Here's how the part is built. I have some questions about the finished solid (model axes, mm). A direction names the side the tool comes from. Round coordinates to 2 decimals unless told otherwise and drop trailing zeros. Loops run counter-clockwise (first coordinate to the right, second up) from the corner with the lowest first, then second, coordinate; pieces in that order, holes last. Notation, with made-up numbers: M 45.25,9 L 102.25,9 A28 ccw 102.25,39 Z; hole C 78,74 d11. An arc over 180 degrees is marked long. Use a Markdown table: item, result.
```python
from build123d import *

# Parameters (mm, degrees)
F1_R      = 11
F1_R_2    = 2.25
F2_DEPTH  = 2
F1_R_3    = 1.75
F3_DEPTH  = 8
F4_DEPTH  = 4.5
F5_DEPTH  = 20
F7_DEPTH  = 24
F9_DEPTH  = 8
F10_R     = 4
F11_DEPTH = 1


with BuildPart() as f2:
    # F1 (on Top) → F2 (new body)
    with BuildSketch(Plane.XY):
        Circle(F1_R)
        Circle(F1_R_2, mode=Mode.SUBTRACT)
    extrude(amount=F2_DEPTH)

    # F1 (on Top) → F3 (join)
    with BuildSketch(Plane.XY):
        Polygon((21.15, 17.15), (17.15, 21.15), (-17.15, 21.15), (-21.15, 17.15), (-21.15, -17.15), (-17.15, -21.15), (17.15, -21.15), (21.15, -17.15), align=None)
        with Locations((-15.5, -15.5)):
            Circle(F1_R_3, mode=Mode.SUBTRACT)
        with Locations((15.5, -15.5)):
            Circle(F1_R_3, mode=Mode.SUBTRACT)
        with Locations((-15.5, 15.5)):
            Circle(F1_R_3, mode=Mode.SUBTRACT)
        Circle(F1_R, mode=Mode.SUBTRACT)
        with Locations((15.5, 15.5)):
            Circle(F1_R_3, mode=Mode.SUBTRACT)
        Circle(F1_R)
        Circle(F1_R_2, mode=Mode.SUBTRACT)
        Circle(F1_R_2)
        with Locations((15.5, -15.5)):
            Circle(F1_R_3)
        with Locations((-15.5, -15.5)):
            Circle(F1_R_3)
        with Locations((-15.5, 15.5)):
            Circle(F1_R_3)
        with Locations((15.5, 15.5)):
            Circle(F1_R_3)
    extrude(amount=-F3_DEPTH)

    # F1 (on Top) → F4 (cut)
    with BuildSketch(Plane.XY):
        with Locations((-15.5, 15.5)):
            Circle(F1_R_3)
        with Locations((15.5, 15.5)):
            Circle(F1_R_3)
        with Locations((15.5, -15.5)):
            Circle(F1_R_3)
        with Locations((-15.5, -15.5)):
            Circle(F1_R_3)
    extrude(amount=-F4_DEPTH, mode=Mode.SUBTRACT)

    # F1 (on Top) → F5 (join)
    with BuildSketch(Plane.XY):
        Circle(F1_R_2)
    extrude(amount=F5_DEPTH)

    # F6 (on face) → F7 (join)
    with BuildSketch(Plane(origin=(0, 0, -8), x_dir=(1, 0, 0), z_dir=(0, 0, -1))):
        Polygon((-13.15, 21.15), (-21.15, 13.15), (-21.15, -13.15), (-13.15, -21.15), (13.15, -21.15), (21.15, -13.15), (21.15, 13.15), (13.15, 21.15), align=None)
    extrude(amount=F7_DEPTH)

    # F8 (on face) → F9 (join)
    with BuildSketch(Plane(origin=(0, 0, -32), x_dir=(1, 0, 0), z_dir=(0, 0, -1))):
        Polygon((-13.15, 21.15), (-17.15, 21.15), (-21.15, 17.15), (-21.15, 13.15), align=None)
        Polygon((13.15, 21.15), (-13.15, 21.15), (-21.15, 13.15), (-21.15, -13.15), (-13.15, -21.15), (13.15, -21.15), (21.15, -13.15), (21.15, 13.15), align=None)
        Polygon((17.15, 21.15), (13.15, 21.15), (21.15, 13.15), (21.15, 17.15), align=None)
        Polygon((21.15, -17.15), (21.15, -13.15), (13.15, -21.15), (17.15, -21.15), align=None)
        Polygon((-13.15, -21.15), (-21.15, -13.15), (-21.15, -17.15), (-17.15, -21.15), align=None)
    extrude(amount=F9_DEPTH)

    # F10 (on face) → F11 (cut)
    with BuildSketch(Plane(origin=(0, 0, -40), x_dir=(1, 0, 0), z_dir=(0, 0, -1))):
        Circle(F10_R)
    extrude(amount=-F11_DEPTH, mode=Mode.SUBTRACT)


solid = f2.part
```
Q1. Will these pins go through, and if not, where does the flat tip stop? P1, Ø1.8, axis at x = 16.5, y = 16.5, coming from the +Z side; P2, Ø12.5, axis at x = 1.5, y = 9.5, coming from the +Z side.
Return value:
| item | result |
|---|---|
| P1 | stops at z = 0 |
| P2 | stops at z = 2 |
Q2. Imagine slicing it at A-A, the plane y = 0. Please give me the cut outline in (x, z).
Return value:
| item | result |
|---|---|
| outline | M -21.15,-40 L -4,-40 L -4,-39 L 4,-39 L 4,-40 L 21.15,-40 L 21.15,0 L 11,0 L 11,2 L 2.25,2 L 2.25,20 L -2.25,20 L -2.25,2 L -11,2 L -11,0 L -21.15,0 Z |
Q3. I need wall thicknesses on line 1 (Y direction, x = 15, z = -1); line 2 (Z direction, x = -18.5, y = 17). Which ranges of each line are inside material? Lowest first, please. Write a range as from..to.
Return value:
| item | result |
|---|---|
| line 1 | y = -21.15..-17.18, -13.82..13.82, 17.18..21.15 |
| line 2 | z = -40..-32, -8..0 |
Q4. We'd pull the mould along Y, two halves only. Please class faces 1 (the cylindrical face through (-0.29, 2.23, 10.87)), 2 (the cylindrical face through (-14.6, -14, -2.2)), 3 (the flat face through (-16, -15, -4.5)), 4 (the flat face through (21.15, 0, -20)): pulls with the +Y half, pulls with the -Y half, needs draft (parallel to the pull), parting line crosses it, or undercut.
Return value:
| item | result |
|---|---|
| face 1 | parting line crosses it |
| face 2 | undercut |
| face 3 | undercut |
| face 4 | needs draft |
Q5. Imagine slicing it at B-B, the plane z = -22.5. Please give me the cut outline in (x, y).
Return value:
| item | result |
|---|---|
| outline | M -21.15,-13.15 L -13.15,-21.15 L 13.15,-21.15 L 21.15,-13.15 L 21.15,13.15 L 13.15,21.15 L -13.15,21.15 L -21.15,13.15 Z |
Q6. Imagine slicing it at C-C, the plane x = -15.5. Please give me the cut outline in (y, z), then the cut area to 3 significant figures.
Return value:
| item | result |
|---|---|
| outline | M -21.15,-40 L 21.15,-40 L 21.15,-32 L 18.8,-32 L 18.8,-8 L 21.15,-8 L 21.15,0 L 17.25,0 L 17.25,-4.5 L 13.75,-4.5 L 13.75,0 L -13.75,0 L -13.75,-4.5 L -17.25,-4.5 L -17.25,0 L -21.15,0 L -21.15,-8 L -18.8,-8 L -18.8,-32 L -21.15,-32 Z |
| area | 1,550 mm^2 |
Q7. For faces 5 (the flat face through (-18, 18, -32)), 6 (the cylindrical face through (-0.867, 3.905, -39.507)), 7 (the flat face through (-18, -18, -32)), 8 (the flat face through (9, -9, 0)), 9 (the flat face through (18, -18, -8)), which set-ups out of +Z, -Z, +X, -X, +Y, -Y let a thin tool reach every point of the face, with its end or its side?
Return value:
| item | result |
|---|---|
| face 5 | -X, +Y |
| face 6 | -Z |
| face 7 | -X, -Y |
| face 8 | +Z |
| face 9 | +X, -Y |
